```python
from build123d import *

# Parameters (mm, degrees)
BASIC_ROD_DEPTH         = 23.01875
BASIC_ROD_DEPTH_BACK    = 23.01875
SKETCH1_R               = 6.35
THEX_DEPTH              = 23.01875
INTERNAL_CUT_DEPTH      = 25.849128119
INTERNAL_CUT_DEPTH_BACK = 25.849128119
SKETCH2_R               = 2.11582
SKETCH9_R               = 4
CUT_EXTRUDE1_DEPTH      = 19.99996
CUT_EXTRUDE2_REACH      = 29.174
CUT_EXTRUDE2_END_RADIUS = 4
SKETCH10_R              = 1.66624


with BuildPart() as part:
    # Sketch1 → Basic Rod (new, two sides: drawn at the far end of the back side and taken through both)
    with BuildSketch(Plane.XY.offset(-BASIC_ROD_DEPTH_BACK)):
        Circle(SKETCH1_R)
    extrude(amount=BASIC_ROD_DEPTH + BASIC_ROD_DEPTH_BACK)

    # Sketch8 → THex (add, symmetric)
    with BuildSketch(Plane.XY):
        with BuildLine():
            Line((-0.888411378, 6.819423871), (-5.461588622, 4.179098758))
            ThreePointArc((-5.461588622, 4.179098758), (-5.955700003, 3.438525), (-6.35, 2.640325113))
            Line((-6.35, 2.640325113), (-6.35, -2.640325113))
            ThreePointArc((-6.35, -2.640325113), (-5.955700003, -3.438525), (-5.461588622, -4.179098758))
            Line((-5.461588622, -4.179098758), (-0.888411378, -6.819423871))
            ThreePointArc((-0.888411378, -6.819423871), (0, -6.87705), (0.888411378, -6.819423871))
            Line((0.888411378, -6.819423871), (5.461588622, -4.179098758))
            ThreePointArc((5.461588622, -4.179098758), (5.955700003, -3.438525), (6.35, -2.640325113))
            Line((6.35, -2.640325113), (6.35, 2.640325113))
            ThreePointArc((6.35, 2.640325113), (5.955700003, 3.438525), (5.461588622, 4.179098758))
            Line((5.461588622, 4.179098758), (0.888411378, 6.819423871))
            ThreePointArc((0.888411378, 6.819423871), (0, 6.87705), (-0.888411378, 6.819423871))
        make_face()
    extrude(amount=THEX_DEPTH, both=True)

    # Sketch2 → Internal Cut (cut, two sides: drawn at the far end of the back side and taken through both)
    with BuildSketch(Plane.XY.offset(-INTERNAL_CUT_DEPTH_BACK)):
        Circle(SKETCH2_R)
    extrude(amount=INTERNAL_CUT_DEPTH + INTERNAL_CUT_DEPTH_BACK, mode=Mode.SUBTRACT)

    # Sketch9 → Cut-Extrude1 (cut)
    with BuildSketch(Plane.XY.offset(23.01875)):
        Circle(SKETCH9_R)
    extrude(amount=-CUT_EXTRUDE1_DEPTH, mode=Mode.SUBTRACT)

    # Cut-Extrude2: up to this cylinder (the profile starts outside it)
    cut_extrude2_end = Plane(origin=(0, 0, 14.01699), z_dir=(0, 0, 1)) * Cylinder(CUT_EXTRUDE2_END_RADIUS, 75.349, mode=Mode.PRIVATE)
    # Sketch10 → Cut-Extrude2 (cut, up to the surface)
    with BuildSketch(Plane.ZY.offset(6.35), mode=Mode.PRIVATE) as cut_extrude2_sk1:
        with Locations((10.01649, 0)):
            Circle(SKETCH10_R)
    cut_extrude2_tool1 = extrude(cut_extrude2_sk1.sketch, amount=-CUT_EXTRUDE2_REACH, mode=Mode.PRIVATE) - cut_extrude2_end
    add(cut_extrude2_tool1.solids().sort_by_distance((-6.35, 0, 10.01649))[0], mode=Mode.SUBTRACT)
    # Sketch10 → Cut-Extrude2 (cut, up to the surface)
    with BuildSketch(Plane.ZY.offset(6.35), mode=Mode.PRIVATE) as cut_extrude2_sk2:
        with Locations((18.01749, 0)):
            Circle(SKETCH10_R)
    cut_extrude2_tool2 = extrude(cut_extrude2_sk2.sketch, amount=-CUT_EXTRUDE2_REACH, mode=Mode.PRIVATE) - cut_extrude2_end
    add(cut_extrude2_tool2.solids().sort_by_distance((-6.35, 0, 18.01749))[0], mode=Mode.SUBTRACT)


solid = part.part
```
Input: part model. Units: mm. Frame: model coordinates. A direction names the side the tool comes from. Coordinates: 2 decimals unless noted, no trailing zeros. Loops run counter-clockwise (first coordinate to the right, second up) from the corner with the lowest first, then second, coordinate; pieces in that order, holes last. Notation, with made-up numbers: M 74,17.5 L 89,17.5 A16 ccw 89,46.5 Z; hole C -30,-37.75 d9. An arc over 180 degrees is marked long. One line per item, written item: value.
(1) Section B-B (z = 7). Output: boundary loops of the cut face in (x, y), and give its area (3 significant figures).
Filled in:
outline: M -6.35,-2.64 A6.88 ccw -5.46,-4.18 L -0.89,-6.82 A6.88 ccw 0.89,-6.82 L 5.46,-4.18 A6.88 ccw 6.35,-2.64 L 6.35,2.64 A6.88 ccw 5.46,4.18 L 0.89,6.82 A6.88 ccw -0.89,6.82 L -5.46,4.18 A6.88 ccw -6.35,2.64 Z; hole C 0,0 d8
area: 87.1 mm^2
(2) Line query: line 1 along Z through (x, y) = (-5.7, 0); line 2 along X through (y, z) = (0, -12); line 3 along Y through (x, z) = (0, 11.5). Output: solid intervals per line, ascending. Write a range as from..to.
Filled in:
line 1: -23.02..8.35, 11.68..16.35, 19.68..23.02
line 2: -6.35..-2.12, 2.12..6.35
line 3: -6.88..-4, 4..6.88
(3) Section A-A (x = 0). Output: boundary loops of the cut face in (y, z), and give its area (3 significant figures).
Filled in:
outline: M -6.88,-23.02 L -2.12,-23.02 L -2.12,3.02 L -4,3.02 L -4,23.02 L -6.88,23.02 Z; M 2.12,-23.02 L 6.88,-23.02 L 6.88,23.02 L 4,23.02 L 4,3.02 L 2.12,3.02 Z
area: 363 mm^2
(4) Section C-C (y = 0). Output: boundary loops of the cut face in (x, z).
Filled in:
outline: M -6.35,-23.02 L -2.12,-23.02 L -2.12,3.02 L -4,3.02 L -4,8.35 L -6.35,8.35 Z; M -6.35,11.68 L -4,11.68 L -4,16.35 L -6.35,16.35 Z; M -6.35,19.68 L -4,19.68 L -4,23.02 L -6.35,23.02 Z; M 2.12,-23.02 L 6.35,-23.02 L 6.35,23.02 L 4,23.02 L 4,3.02 L 2.12,3.02 Z
(5) Section D-D (z = -5.5). Output: boundary loops of the cut face in (x, y).
Filled in:
outline: M -6.35,-2.64 A6.88 ccw -5.46,-4.18 L -0.89,-6.82 A6.88 ccw 0.89,-6.82 L 5.46,-4.18 A6.88 ccw 6.35,-2.64 L 6.35,2.64 A6.88 ccw 5.46,4.18 L 0.89,6.82 A6.88 ccw -0.89,6.82 L -5.46,4.18 A6.88 ccw -6.35,2.64 Z; hole C 0,0 d4.23
(6) Pin query (flat end, axial travel): pin 1 (2.5 mm diameter, centred on y = 0, z = 10.02, fed in from -X); pin 2 (5 mm diameter, centred on x = 0, y = 0, fed in from +Z); pin 3 (3 mm diameter, centred on x = 1, z = 0.5, fed in from +Y). Return the tip coordinate at first contact, or that it passes through.
Filled in:
pin 1: x = 3.8
pin 2: z = 3.02
pin 3: y = 6.88
(7) Pull-direction query (Y, two-part tool) for faces 4 (the cylindrical face through (-5.012, 0.5, 11.606)), 5 (the cylindrical face through (-5.95, 3.45, 0.32)), 6 (the flat face through (-6.35, 0, 0)); classes: +Y half, -Y half, draft (parallel to the pull), parting line (faces both ways), or undercut.
Filled in:
face 4: undercut
face 5: +Y half
face 6: draft
(8) Reachability of faces 1 (the cylindrical face through (-5.012, 0.5, 19.607)), 2 (the flat face through (3.21, 5.48, 0.32)), 3 (the cylindrical face through (3.695, -1.532, 13.159)) from +Z, -Z, +X, -X, +Y, -Y: full face, straight path, thin tool, end or side. Return the list, or none.
Filled in:
face 1: -X
face 2: +Z, -Z, +X, +Y
face 3: +Z
